Geometry: final body of the model. Coordinates: model frame, mm. Face numbers are marked on the shaded views. A direction names the side the tool comes from. Give positions to 0.01 mm unless a question says otherwise; leave off trailing zeros. Write each loop counter-clockwise with the first axis right and the second up, starting at its lowest first coordinate (ties: lowest second). Pieces come first, ordered by that corner, then holes. Notation, with made-up numbers: M 52,-22 L 84,-22 A27 cw 84,14 Z; hole C -27.5,31 d6. An arc over 180 degrees is marked long. Use a Markdown table: item, result. Add a question column.
1) Set-up query: the marked faces 1, 2 and 3. Return all of +Z, -Z, +X, -X, +Y, -Y with unobstructed straight access to the full face (end or side cutting, diameter ignored); none if empty.
2) Draft query along Z for the marked faces 4, 5 and 6. Return one class per face: +Z half, -Z half, draft (parallel to the pull), parting line (faces both ways), or undercut.
3) Section B-B on y = 4. Return the cut outline in (x, z), then the cut area to 3 significant figures.
4) Line query: line 1 (Z direction, x = 25.4, y = 2.75); line 2 (X direction, y = 5.25, z = -12.5); line 3 (Z direction, x = 27, y = 2.75). Output: solid intervals per line, ascending.
5) Section A-A on x = 25.4. Return the cut outline in (y, z).
6) Section C-C on x = 37.5. Return the cut outline in (y, z).
7) Pin query (flat end, axial travel): pin 1 (1 mm diameter, centred on x = 23.5, z = -23, fed in from -Y); pin 2 (3 mm diameter, centred on y = 4.5, z = -34, fed in from +X); pin 3 (3 mm diameter, centred on x = 13, y = 3, fed in from -Z); pin 4 (3 mm diameter, centred on y = 4.5, z = -34, fed in from -X). Return the tip coordinate at first contact, or that it passes through.
```python
from build123d import *

# Parameters (mm, degrees)
SKETCH2_R           = 0.840105
SKETCH2_R_2         = 1.016
BOSS_EXTRUDE2_DEPTH = 6.35


with BuildPart() as part:
    # Sketch2 → Boss-Extrude2 (new body)
    with BuildSketch(Plane(origin=(0, 0, 0), x_dir=(1, 0, 0), z_dir=(0, 1, 0))):
        with BuildLine():
            Line((19.05, -6.35), (31.75, -6.35))
            ThreePointArc((31.75, -6.35), (45.220384182, -0.770384182), (50.8, 12.7))
            Line((50.8, 12.7), (50.8, 21.59))
            ThreePointArc((50.8, 21.59), (49.353345536, 27.604748069), (45.329825459, 32.303821346))
            Line((45.329825459, 32.303821346), (31.75, 32.303821346))
            Line((31.75, 32.303821346), (31.75, 34.843821346))
            Line((31.75, 34.843821346), (29.21, 34.843821346))
            Line((29.21, 34.843821346), (29.21, 32.303821346))
            Line((29.21, 32.303821346), (26.67, 32.303821346))
            Line((26.67, 32.303821346), (26.67, 34.843821346))
            Line((26.67, 34.843821346), (24.13, 34.843821346))
            Line((24.13, 34.843821346), (24.13, 32.303821346))
            Line((24.13, 32.303821346), (21.59, 32.303821346))
            Line((21.59, 32.303821346), (21.59, 34.843821346))
            Line((21.59, 34.843821346), (19.05, 34.843821346))
            Line((19.05, 34.843821346), (19.05, 32.303821346))
            Line((19.05, 32.303821346), (5.470174541, 32.303821346))
            ThreePointArc((5.470174541, 32.303821346), (1.446654464, 27.604748069), (0, 21.59))
            Line((0, 21.59), (0, 12.7))
            ThreePointArc((0, 12.7), (5.579615818, -0.770384182), (19.05, -6.35))
        make_face()
        with Locations((45.329825459, 28.017571346)):
            Circle(SKETCH2_R, mode=Mode.SUBTRACT)
        with Locations((25.4, 26.983791346)):
            Circle(SKETCH2_R_2, mode=Mode.SUBTRACT)
        with Locations((5.47017448, 28.017571346)):
            Circle(SKETCH2_R, mode=Mode.SUBTRACT)
        with Locations((25.4, -0.730148654)):
            Circle(SKETCH2_R_2, mode=Mode.SUBTRACT)
        Polygon((25.4, 24.683821346), (31.369, 24.683821346), (31.369, 1.569821346), (19.431, 1.569821346), (19.431, 24.683821346), align=None, mode=Mode.SUBTRACT)
    extrude(amount=BOSS_EXTRUDE2_DEPTH)


solid = part.part
```
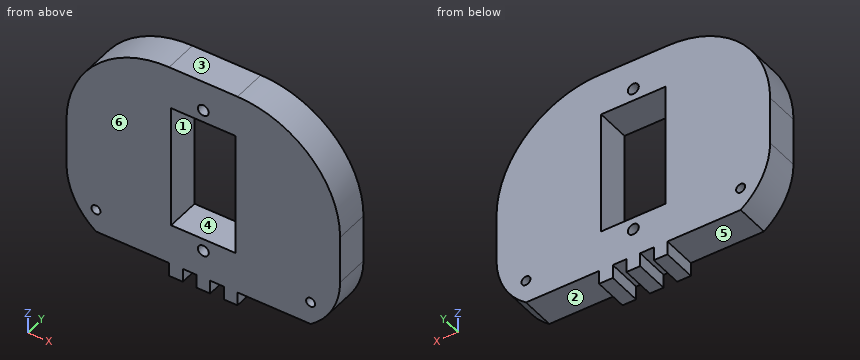
Found:
| question | item | result |
|---|---|---|
| 1 | face 1 | +Y, -Y |
| 1 | face 2 | -Z, +X, +Y, -Y |
| 1 | face 3 | +Z, +X, -X, +Y, -Y |
| 2 | face 4 | undercut |
| 2 | face 5 | -Z half |
| 2 | face 6 | draft |
| 3 | outline | M 0,-21.59 A13.23 ccw 5.47,-32.3 L 19.05,-32.3 L 19.05,-34.84 L 21.59,-34.84 L 21.59,-32.3 L 24.13,-32.3 L 24.13,-34.84 L 26.67,-34.84 L 26.67,-32.3 L 29.21,-32.3 L 29.21,-34.84 L 31.75,-34.84 L 31.75,-32.3 L 45.33,-32.3 A13.23 ccw 50.8,-21.59 L 50.8,-12.7 A19.05 ccw 31.75,6.35 L 19.05,6.35 A19.05 ccw 0,-12.7 Z; hole C 5.47,-28.02 d1.68; hole M 19.43,-24.68 L 31.37,-24.68 L 31.37,-1.57 L 19.43,-1.57 Z; hole C 25.4,-26.98 d2.03; hole C 25.4,0.73 d2.03; hole C 45.33,-28.02 d1.68 |
| 3 | area | 1,510 mm² |
| 4 | line 1 | -34.84 to -28, -25.97 to -24.68, -1.57 to -0.29, 1.75 to 6.35 |
| 4 | line 2 | 0 to 19.43, 31.37 to 50.8 |
| 4 | line 3 | -32.3 to -24.68, -1.57 to 6.35 |
| 5 | outline | M 0,-34.84 L 6.35,-34.84 L 6.35,-28 L 0,-28 Z; M 0,-25.97 L 6.35,-25.97 L 6.35,-24.68 L 0,-24.68 Z; M 0,-1.57 L 6.35,-1.57 L 6.35,-0.29 L 0,-0.29 Z; M 0,1.75 L 6.35,1.75 L 6.35,6.35 L 0,6.35 Z |
| 6 | outline | M 0,-32.3 L 6.35,-32.3 L 6.35,5.46 L 0,5.46 Z |
| 7 | pin 1 | through |
| 7 | pin 2 | x = 31.75 |
| 7 | pin 3 | z = -32.3 |
| 7 | pin 4 | x = 19.05 |
